```python
from build123d import *

# Parameters (mm, degrees)
SKETCH1_R           = 55
BOSS_EXTRUDE1_DEPTH = 20
SKETCH9_W           = 40
SKETCH9_H           = 20
BOSS_EXTRUDE4_DEPTH = 20
SKETCH11_R          = 4.1
CUT_EXTRUDE6_DEPTH  = 21
SKETCH12_R          = 52
CUT_EXTRUDE7_DEPTH  = 17
BOSS_EXTRUDE5_DEPTH = 17
SKETCH14_W          = 12.8
SKETCH14_H          = 15
CUT_EXTRUDE8_DEPTH  = 39.466128658
SKETCH16_W          = 35
SKETCH16_H          = 15
CUT_EXTRUDE9_DEPTH  = 10
CHAMFER1_SIZE       = 1
CHAMFER1_SIZE2      = 2.747477419


with BuildPart() as part:
    # Sketch1 → Boss-Extrude1 (new body)
    with BuildSketch(Plane(origin=(0, 0, 0), x_dir=(1, 0, 0), z_dir=(0, 1, 0))):
        with Locations(Location((0, 0, 0), (0, 0, 270))):  # turned: the seam where the file's is
            Circle(SKETCH1_R)
    extrude(amount=BOSS_EXTRUDE1_DEPTH)

    # Sketch9 → Boss-Extrude4 (add)
    with BuildSketch(Plane.XZ):
        with Locations((0, 61.23475383)):
            Rectangle(SKETCH9_W, SKETCH9_H)
    extrude(amount=-BOSS_EXTRUDE4_DEPTH)

    # Sketch11 → Cut-Extrude6 (cut, through all)
    with BuildSketch(Plane(origin=(0, 20, 0), x_dir=(1, 0, 0), z_dir=(0, 1, 0))):
        with Locations(Location((-10, -61.23475383, 0), (0, 0, 270))):  # turned: the seam where the file's is
            Circle(SKETCH11_R)
        with Locations(Location((10, -61.23475383, 0), (0, 0, 270))):  # turned: the seam where the file's is
            Circle(SKETCH11_R)
    extrude(amount=-CUT_EXTRUDE6_DEPTH, mode=Mode.SUBTRACT)

    # Sketch12 → Cut-Extrude7 (cut)
    with BuildSketch(Plane.XZ):
        with Locations(Location((0, 0, 0), (0, 0, 270))):  # turned: the seam where the file's is
            Circle(SKETCH12_R)
    extrude(amount=-CUT_EXTRUDE7_DEPTH, mode=Mode.SUBTRACT)

    # Sketch13 → Boss-Extrude5 (add)
    with BuildSketch(Plane.XZ):
        Polygon((-27.329455823, 44.239132501), (-38.821330473, 34.596304721), (-36.242802171, 41.369787173), align=None)
    extrude(amount=-BOSS_EXTRUDE5_DEPTH)

    # Sketch14 → Cut-Extrude8 (cut, through all)
    with BuildSketch(Plane(origin=(-33.075393148, 0, 39.417718611), x_dir=(-0.766044443, 0, -0.64278761), z_dir=(0.64278761, 0, -0.766044443))):
        with Locations((0, 8.5)):
            Rectangle(SKETCH14_W, SKETCH14_H)
    extrude(amount=-CUT_EXTRUDE8_DEPTH, mode=Mode.SUBTRACT)

    # Sketch16 → Cut-Extrude9 (cut)
    with BuildSketch(Plane.XZ):
        with Locations((0, 61.23475383)):
            Rectangle(SKETCH16_W, SKETCH16_H)
    extrude(amount=-CUT_EXTRUDE9_DEPTH, mode=Mode.SUBTRACT)

    # Chamfer1
    chamfer1_edges = [part.edges().sort_by_distance(p)[0] for p in [
        (17.5, 0, 61.23475383),
        (0, 0, 68.73475383),
        (-17.5, 0, 61.23475383),
        (0, 0, 53.73475383),
    ]]
    chamfer1_side = [part.faces().sort_by_distance(p)[0] for p in [
        (-18.325628086, 0, 61.23475383),
    ]]
    chamfer(chamfer1_edges, length=CHAMFER1_SIZE, length2=CHAMFER1_SIZE2, reference=chamfer1_side[0])


solid = part.part
```
For this review, take the finished solid that the model builds, in its own axes (mm). A direction names the side the tool comes from. Give positions to 0.01 mm unless a question says otherwise; leave off trailing zeros. Write each loop counter-clockwise with the first axis right and the second up, starting at its lowest first coordinate (ties: lowest second). Pieces come first, ordered by that corner, then holes. Notation, with made-up numbers: M -27.75,-26 L -3.75,-26 A27 ccw -3.75,8 Z; hole C 87.25,75 d8. An arc over 180 degrees is marked long. Answer as a JSON object with one key per item and string values. Group by question number.
Item 1: Consider section D-D on x = 37.5. Write out the cut boundary in (y, z), plus the area to 3 significant figures.
Item 2: Draft analysis for pull direction Y (two halves, no side actions). For faces 4 (the flat face through (0, 6, 53.735)), 5 (the flat face through (0.3, 0, -52.4)), 6 (the flat face through (-34, 1, 41)), state which applies: +Y half, -Y half, draft (parallel to the pull), parting line (faces both ways), or undercut.
Item 3: Consider section A-A on y = 5.75. Write out the cut boundary in (x, z), plus the area to 3 significant figures.
Item 4: Consider section B-B on x = 10. Write out the cut boundary in (y, z), plus the area to 3 significant figures.
Item 5: Consider section C-C on z = 0. Write out the cut boundary in (x, y).
Item 6: For pin 1 Ø3.5 at (y, z) = (7, 63.5) entering from -X; pin 2 Ø8 at (x, y) = (-18.5, 10) entering from -Z; pin 3 Ø6 at (y, z) = (8.5, 39.5) entering from -X, all flat-tipped, find the tip position at first contact; note any pin that passes through.
Item 7: Tool access review of faces 1 (the flat face through (-20, 10, 61)), 2 (the flat face through (1, 17, 1)), 3 (the cylindrical face through (8.43, 15.07, 65.022)): name each direction out of +Z, -Z, +X, -X, +Y, -Y from which nothing blocks a thin tool from reaching the whole face with its end or side.
Item 8: For probe 1 along X at (y, z) = (10.75, 0); probe 2 along X at (y, z) = (13.75, 63.5); probe 3 along Z at (x, y) = (11.5, 15), list the stretches that pass through material, from the lowest coordinate up. Write a range as [from, to].
Check result:
{
 "1": {"outline": "M 0,-40.23 L 20,-40.23 L 20,40.23 L 0,40.23 L 0,36.02 L 17,36.02 L 17,-36.02 L 0,-36.02 Z", "area": "385 mm^2"},
 "2": {"face 4": "draft", "face 5": "-Y half", "face 6": "undercut"},
 "3": {"outline": "M -40.02,37.73 A55 ccw long 20,51.23 L 20,71.23 L -20,71.23 L -20,51.23 A55 ccw -30.21,45.96 L -28.17,43.53 L -27.33,44.24 A52 cw long -38.82,34.6 L -37.98,35.3 Z; hole M -17.5,53.73 L 17.5,53.73 L 17.5,68.73 L -17.5,68.73 Z", "area": "1,140 mm^2"},
 "4": {"outline": "M 0,-54.08 L 20,-54.08 L 20,57.13 L 10,57.13 L 10,53.73 L 2.75,53.73 L 0,52.73 L 0,51.03 L 17,51.03 L 17,-51.03 L 0,-51.03 Z; M 0,69.73 L 2.75,68.73 L 10,68.73 L 10,65.33 L 20,65.33 L 20,71.23 L 0,71.23 Z", "area": "537 mm^2"},
 "5": {"outline": "M -55,0 L -52,0 L -52,17 L 52,17 L 52,0 L 55,0 L 55,20 L -55,20 Z"},
 "6": {"pin 1": "stops at x = -20", "pin 2": "stops at z = -53.05", "pin 3": "stops at x = -41.14"},
 "7": {"face 1": "+Z, -X, +Y, -Y", "face 2": "-Y", "face 3": "+Y, -Y"},
 "8": {"probe 1": "x = [-55, -52], [52, 55]", "probe 2": "x = [-20, -13.42], [-6.58, 6.58], [13.42, 20]", "probe 3": "z = [-53.78, -50.71], [50.71, 57.42], [65.05, 71.23]"}
}
